Could you check a few things on this model? Use its own coordinates, in mm. Coordinates: 2 decimals unless noted, no trailing zeros. Order: outer loops, then holes, each group sorted by start corner. A loop starts at its lowest first (then second) coordinate and runs counter-clockwise, first axis right, second up. Notation, with made-up numbers: (76, 25.5) - (95, 25.5) arc R17 ccw to (95, 56.5) - close; hole circle Ø3 at (32, -15.5). An arc over 180 degrees is marked (long way). Answer as CSV lines item,"result". Start each with the question number.
1. I want a section at A-A, the plane x = 7.25. List the corners of the cut face in (y, z) for me.
2. For pin 1 (3 mm diameter, centred on x = 13, y = 18.5, fed in from +Z); pin 2 (1.5 mm diameter, centred on y = 122.5, z = 15.5, fed in from -X); pin 3 (2 mm diameter, centred on x = 7.5, y = 43.5, fed in from +Z), each with a flat end and sliding along its axis, tell me the tip position at first contact or that it passes through.
3. I want a section at B-B, the plane y = 93. List the corners of the cut face in (x, z) for me, and give its area (3 significant figures).
4. I need wall thicknesses on probe 1 along X at (y, z) = (240, 2); probe 2 along Y at (x, z) = (-3.25, 11); probe 3 along Y at (x, z) = (-2.5, 1.3). Which ranges of each line are inside material? Lowest first, please.
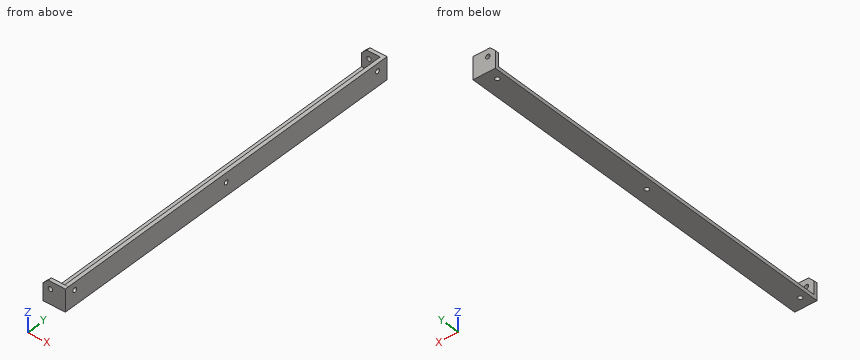
from build123d import *

# Parameters (mm, degrees)
SKETCH1_W           = 25
SKETCH1_H           = 500
SKETCH1_R           = 3
BOSS_EXTRUDE1_DEPTH = 5
SKETCH2_W           = 5
SKETCH2_H           = 500
BOSS_EXTRUDE2_DEPTH = 30
SKETCH3_R           = 3
CUT_EXTRUDE1_DEPTH  = 20.5
SKETCH4_R           = 3
BOSS_EXTRUDE3_DEPTH = 5
SKETCH5_R           = 3
BOSS_EXTRUDE4_DEPTH = 5


with BuildPart() as part:
    # Sketch1 → Boss-Extrude1 (new body)
    with BuildSketch(Plane.XY):
        Rectangle(SKETCH1_W, SKETCH1_H)
        with Locations((-2.5, 240)):
            Circle(SKETCH1_R, mode=Mode.SUBTRACT)
        with Locations((-2.5, -240)):
            Circle(SKETCH1_R, mode=Mode.SUBTRACT)
        Circle(SKETCH1_R, mode=Mode.SUBTRACT)
    extrude(amount=BOSS_EXTRUDE1_DEPTH)

    # Sketch2 → Boss-Extrude2 (add)
    with BuildSketch(Plane(origin=(0, 0, 0), x_dir=(-1, 0, 0), z_dir=(0, 0, -1))):
        with Locations((-15, 0)):
            Rectangle(SKETCH2_W, SKETCH2_H)
    extrude(amount=-BOSS_EXTRUDE2_DEPTH)

    # Sketch3 → Cut-Extrude1 (cut)
    with BuildSketch(Plane.ZY.offset(-12.5)):
        with Locations((20, -240)):
            Circle(SKETCH3_R)
        with Locations((17.5, 0)):
            Circle(SKETCH3_R)
        with Locations((20, 240)):
            Circle(SKETCH3_R)
    extrude(amount=-CUT_EXTRUDE1_DEPTH, mode=Mode.SUBTRACT)

    # Sketch4 → Boss-Extrude3 (add)
    with BuildSketch(Plane(origin=(0, 250, 0), x_dir=(1, 0, 0), z_dir=(0, 1, 0))):
        Polygon((-12.5, 0), (17.5, 0), (17.5, -30), (-5.428932188, -30), (-12.5, -22.928932188), align=None)
        with Locations((-2.5, -20)):
            Circle(SKETCH4_R, mode=Mode.SUBTRACT)
    extrude(amount=BOSS_EXTRUDE3_DEPTH)

    # Sketch5 → Boss-Extrude4 (add)
    with BuildSketch(Plane(origin=(0, -250, 0), x_dir=(-1, 0, 0), z_dir=(0, -1, 0))):
        Polygon((12.5, 0), (-17.5, 0), (-17.5, -30), (5.456313249, -30.054721724), (12.5, -22.95637847), align=None)
        with Locations((2.5, -20)):
            Circle(SKETCH5_R, mode=Mode.SUBTRACT)
    extrude(amount=BOSS_EXTRUDE4_DEPTH)


solid = part.part
Solved:
1,outline,"(-255, 0) - (255, 0) - (255, 30) - (250, 30) - (250, 5) - (-250, 5) - (-250, 30.02) - (-255, 30.02) - close"
2,pin 1,"stops at z = 30"
2,pin 2,"stops at x = 12.5"
2,pin 3,"stops at z = 5"
3,outline,"(-12.5, 0) - (17.5, 0) - (17.5, 30) - (12.5, 30) - (12.5, 5) - (-12.5, 5) - close"
3,area,"275 mm2"
4,probe 1,"x = -12.5 to -5.5, 0.5 to 17.5"
4,probe 2,"y = -255 to -250, 250 to 255"
4,probe 3,"y = -255 to -243, -237 to -1.66, 1.66 to 237, 243 to 255"
